from build123d import *

# Parameters (mm, degrees)
F0_W     = 25
F0_H     = 45
F0_R     = 1.75
F1_DEPTH = 3
F2_R     = 5


with BuildPart() as f1:
    # F0 (on Top) → F1 (new body)
    with BuildSketch(Plane.XY):
        with Locations((-2.834506, 15.854306)):
            Rectangle(F0_W, F0_H)
        with Locations((-10.334506, -1.645694)):
            Circle(F0_R, mode=Mode.SUBTRACT)
        with Locations((4.665494, -1.645694)):
            Circle(F0_R, mode=Mode.SUBTRACT)
    extrude(amount=F1_DEPTH)

    # F2
    f2_edges = [f1.edges().sort_by_distance(p)[0] for p in [
        (9.665494, 38.354306, 1.5),
        (-15.334506, 38.354306, 1.5),
    ]]
    fillet(f2_edges, radius=F2_R)


solid = f1.part
Can you work these out from the model? Positions are in its coordinate system, mm. Round coordinates to 2 decimals unless told otherwise and drop trailing zeros. Loops run counter-clockwise (first coordinate to the right, second up) from the corner with the lowest first, then second, coordinate; pieces in that order, holes last. Notation, with made-up numbers: (11.25, -26.75) - (66.25, -26.75) arc R13 ccw to (66.25, -16.75) - close; hole circle Ø10 at (-19.75, 80). An arc over 180 degrees is marked (long way). Answer in a Markdown table with one row per item. Add a question column.
Q1. We'd pull the mould along X, two halves only. Please class faces 1 (the cylindrical face through (-13.91, 36.85, 1.52)), 2 (the cylindrical face through (6.28, -2.32, 1.48)), 3 (the flat face through (-3, -6.646, 1)): pulls with the +X half, pulls with the -X half, needs draft (parallel to the pull), parting line crosses it, or undercut.
Q2. I want a section at C-C on x = 7.5. List the corners of the cut face in (y, z) for me, and give its area (3 significant figures).
Q3. For pin 1 Ø4.5 at (x, y) = (-10.33, -1.65) entering from -Z; pin 2 Ø3 at (x, y) = (4.67, -1.65) entering from +Z, each with a flat end and sliding along its axis, tell me the tip position at first contact or that it passes through.
Q4. I need wall thicknesses on L1, parallel to Y at x = 6, z = 2.3; L2, parallel to Y at x = -10.75, z = 1.5; L3, parallel to X at y = 36, z = 0.35. Which ranges of each line are inside material? Lowest first, please.
Q5. I want a section at B-B on z = 0.5. List the corners of the cut face in (x, y) for me.
Q6. I want a section at A-A on y = -1. List the corners of the cut face in (x, z) for me.
A:
| question | item | result |
|---|---|---|
| 1 | face 1 | pulls with the -X half |
| 1 | face 2 | undercut |
| 1 | face 3 | needs draft |
| 2 | outline | (-6.65, 0) - (37.47, 0) - (37.47, 3) - (-6.65, 3) - close |
| 2 | area | 132 mm^2 |
| 3 | pin 1 | z = 0 |
| 3 | pin 2 | through |
| 4 | L1 | -6.65 to -2.78, -0.51 to 38.17 |
| 4 | L2 | -6.65 to -3.35, 0.05 to 38.34 |
| 4 | L3 | -14.58 to 8.91 |
| 5 | outline | (-15.33, -6.65) - (9.67, -6.65) - (9.67, 33.35) arc R5 ccw to (4.67, 38.35) - (-10.33, 38.35) arc R5 ccw to (-15.33, 33.35) - close; hole circle Ø3.5 at (-10.33, -1.65); hole circle Ø3.5 at (4.67, -1.65) |
| 6 | outline | (-15.33, 0) - (-11.96, 0) - (-11.96, 3) - (-15.33, 3) - close; (-8.71, 0) - (3.04, 0) - (3.04, 3) - (-8.71, 3) - close; (6.29, 0) - (9.67, 0) - (9.67, 3) - (6.29, 3) - close |
